For this review, take the finished solid that the model builds, in its own axes (mm). Face numbers are marked on the shaded views. Round coordinates to 2 decimals unless told otherwise and drop trailing zeros. Loops run counter-clockwise (first coordinate to the right, second up) from the corner with the lowest first, then second, coordinate; pieces in that order, holes last. Notation, with made-up numbers: M 25.5,-8.75 L 68.5,-8.75 A21 ccw 68.5,7.25 Z; hole C 45,7.5 d6. An arc over 180 degrees is marked long. One line per question, with ' | ' between items. Start each with the question number.
1) For probe 1 along Y at (x, z) = (54, -9); probe 2 along Y at (x, z) = (56.5, -36); probe 3 along X at (y, z) = (71, -3), list the stretches that pass through material, from the lowest coordinate up. Write a range as from..to.
2) For pin 1 Ø3 at (x, y) = (48.5, 46) entering from -Z; pin 2 Ø5.5 at (x, z) = (8.5, -15.5) entering from -Y, all flat-tipped, find the tip position at first contact; note any pin that passes through.
3) We need section C-C (y = 67). Give the boundary of the cut face in (x, z).
4) We need section A-A (z = -34.5). Give the boundary of the cut face in (x, y).
5) We need section B-B (x = 53). Give the boundary of the cut face in (y, z), and give its area (3 significant figures).
6) We need section D-D (x = 39). Give the boundary of the cut face in (y, z), and give its area (3 significant figures).
7) Mouldability with a two-part tool opening along X and no side actions: class the marked faces 1, 2 and 3 as pulls with the +X half, pulls with the -X half, needs draft (parallel to the pull), parting line crosses it, or undercut.
```python
from build123d import *

# Parameters (mm, degrees)
ESQUISSE2_W        = 60
ESQUISSE2_H        = 80
BOSS_EXTRU_1_DEPTH = 2
BOSS_EXTRU_3_DEPTH = 40


with BuildPart() as part:
    # Esquisse2 → Boss.-Extru.1 (new body)
    with BuildSketch(Plane.XY):
        with Locations((30, 40)):
            Rectangle(ESQUISSE2_W, ESQUISSE2_H)
    extrude(amount=BOSS_EXTRU_1_DEPTH)

    # Esquisse3 → Boss.-Extru.3 (add)
    with BuildSketch(Plane(origin=(0, 0, 0), x_dir=(-1, 0, 0), z_dir=(0, 0, -1))):
        Polygon((-60, 0), (-50, 0), (-50, 5), (-55, 5), (-55, 10), (-60, 10), align=None)
        Polygon((0, 0), (-10, 0), (-10, 5), (-5, 5), (-5, 10), (0, 10), align=None)
        Polygon((0, 80), (-10, 80), (-10, 75), (-5, 75), (-5, 70), (0, 70), align=None)
        Polygon((-60, 80), (-50, 80), (-50, 75), (-55, 75), (-55, 70), (-60, 70), align=None)
    extrude(amount=BOSS_EXTRU_3_DEPTH)


solid = part.part
```
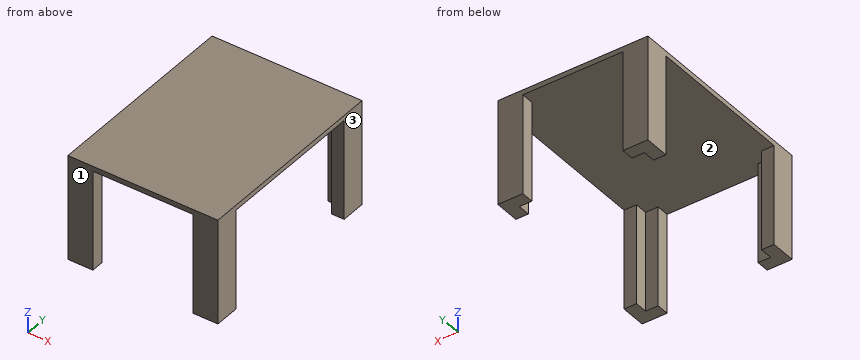
Answers below:
1) probe 1: 0..5, 75..80 | probe 2: 0..10, 70..80 | probe 3: 0..5, 55..60
2) pin 1: z = 0 | pin 2: y = 0
3) outline: M 0,0 L 60,0 L 60,2 L 0,2 Z
4) outline: M 0,0 L 10,0 L 10,5 L 5,5 L 5,10 L 0,10 Z; M 0,70 L 5,70 L 5,75 L 10,75 L 10,80 L 0,80 Z; M 50,0 L 60,0 L 60,10 L 55,10 L 55,5 L 50,5 Z; M 50,75 L 55,75 L 55,70 L 60,70 L 60,80 L 50,80 Z
5) outline: M 0,-40 L 5,-40 L 5,0 L 75,0 L 75,-40 L 80,-40 L 80,2 L 0,2 Z | area: 560 mm^2
6) outline: M 0,0 L 80,0 L 80,2 L 0,2 Z | area: 160 mm^2
7) face 1: needs draft | face 2: undercut | face 3: pulls with the +X half
